For this review, use the dimensioned drawing (mm, ordinates from the lowest corner) and the shaded views. Coordinates: 2 decimals unless noted, no trailing zeros. Order: outer loops, then holes, each group sorted by start corner. A loop starts at its lowest first (then second) coordinate and runs counter-clockwise, first axis right, second up. Notation, with made-up numbers: (53, 3.5) -> (108, 3.5) arc R15 cw to (108, 14.5) -> close; hole circle Ø4 at (-7.75, 28). An arc over 180 degrees is marked (long way). Use one line per item in the form item = value. Start each with the question number.
(1) Take a section at C-C (x = 2.25). State the section outline as (y, z) points.
(2) Take a section at D-D (y = 10). State the section outline as (x, z) points, then the cut area to 3 significant figures.
(3) Take a section at A-A (y = 25). State the section outline as (x, z) points, then the cut area to 3 significant figures.
(4) Wall thickness on line 1 along Y through (x, z) = (1.15, 25); line 2 along Y through (x, z) = (0.2, 20.5); line 3 along Z through (x, y) = (0.7, 29): over which ranges is each line inside the solid? List them lowest first.
(5) Insertion check: pin 1 Ø1.5 at (x, y) = (0.5, 39) entering from -Z; pin 2 Ø1.5 at (x, z) = (0.5, 27) entering from -Y. Each pin has a flat end and moves straight along its axis. Give the tip position at first contact, or say it passes through.
(6) Mouldability with a two-part tool opening along Y and no side actions: class the marked faces 1, 2 and 3 as +Y half, -Y half, draft (parallel to the pull), parting line (faces both ways), or undercut.
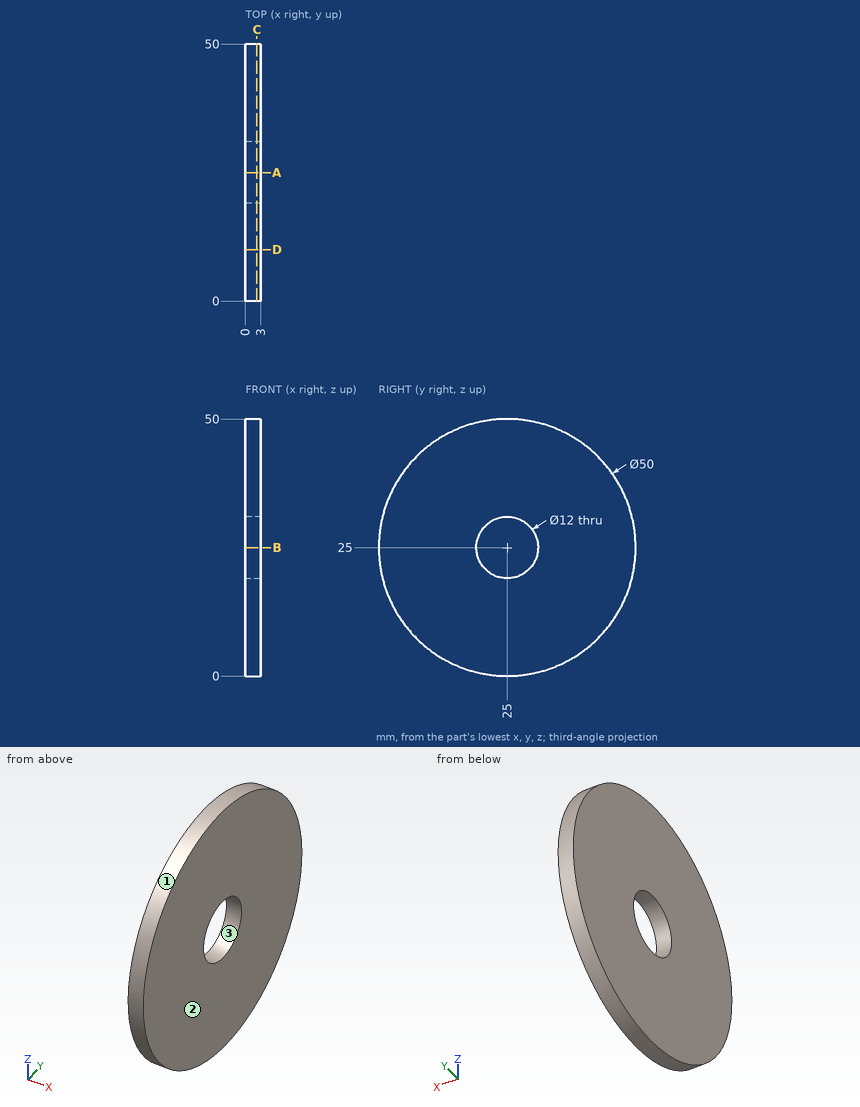
Findings:
q1.outline = circle Ø50 at (25, 25); hole circle Ø12 at (25, 25)
q2.outline = (0, 5) -> (3, 5) -> (3, 45) -> (0, 45) -> close
q2.area = 120 mm²
q3.outline = (0, 0) -> (3, 0) -> (3, 19) -> (0, 19) -> close; (0, 31) -> (3, 31) -> (3, 50) -> (0, 50) -> close
q3.area = 114 mm²
q4.line_1 = 0 to 19, 31 to 50
q4.line_2 = 0.41 to 21.03, 28.97 to 49.59
q4.line_3 = 0.32 to 20.53, 29.47 to 49.68
q5.pin_1 = 3.8
q5.pin_2 = 0.03
q6.face_1 = parting line
q6.face_2 = draft
q6.face_3 = undercut
